from build123d import *

# Parameters (mm, degrees)
SKETCH7_W               = 120
SKETCH7_H               = 30
BOSS_EXTRUDE4_DEPTH     = 100
SKETCH8_W               = 20
SKETCH8_H               = 100
BOSS_EXTRUDE5_DEPTH     = 40
SKETCH9_W               = 100
SKETCH9_H               = 20
BOSS_EXTRUDE6_DEPTH     = 40
CUT_EXTRUDE2_DEPTH      = 99.261072461
CUT_EXTRUDE2_DEPTH_BACK = 40
SKETCH11_R              = 10
CUT_EXTRUDE3_DEPTH      = 120
SKETCH12_W              = 4
SKETCH12_H              = 16
SKETCH12_H_2            = 4
SKETCH12_W_2            = 16
SKETCH12_W_3            = 20
SKETCH12_H_3            = 20
BOSS_EXTRUDE7_DEPTH     = 30


with BuildPart() as part:
    # Sketch7 → Boss-Extrude4 (new body)
    with BuildSketch(Plane.XY):
        with Locations((0.090771558, -5.559757943)):
            Rectangle(SKETCH7_W, SKETCH7_H)
    extrude(amount=-BOSS_EXTRUDE4_DEPTH)

    # Sketch8 → Boss-Extrude5 (add)
    with BuildSketch(Plane(origin=(0, 9.440242057, 0), x_dir=(1, 0, 0), z_dir=(0, 1, 0))):
        with Locations((-49.909228442, 50)):
            Rectangle(SKETCH8_W, SKETCH8_H)
    extrude(amount=BOSS_EXTRUDE5_DEPTH)

    # Sketch9 → Boss-Extrude6 (add)
    with BuildSketch(Plane(origin=(0, 9.440242057, 0), x_dir=(1, 0, 0), z_dir=(0, 1, 0))):
        with Locations((10.090771558, 50)):
            Rectangle(SKETCH9_W, SKETCH9_H)
    extrude(amount=BOSS_EXTRUDE6_DEPTH)

    # Sketch10 → Cut-Extrude2 (cut, two sides: drawn at the far end of the back side and taken through both)
    with BuildSketch(Plane.XY.offset(-40).offset(-CUT_EXTRUDE2_DEPTH_BACK)):
        Polygon((-284.082083156, 147.109383943), (-39.909228442, 49.440242057), (60.090771558, 9.440242057), (304.263626273, -88.228899828), (499.601910045, 400.116809601), (-88.743799385, 635.455093373), align=None)
    extrude(amount=CUT_EXTRUDE2_DEPTH + CUT_EXTRUDE2_DEPTH_BACK, mode=Mode.SUBTRACT)

    # Sketch11 → Cut-Extrude3 (cut)
    with BuildSketch(Plane(origin=(60.090771558, 0, 0), x_dir=(0, 0, -1), z_dir=(1, 0, 0))):
        with Locations(Location((50, -5.559757943, 0), (0, 0, 90))):
            Circle(SKETCH11_R)
    extrude(amount=-CUT_EXTRUDE3_DEPTH, mode=Mode.SUBTRACT)

    # Sketch12 → Boss-Extrude7 (add)
    with BuildSketch(Plane.XZ.offset(20.559757943)):
        with Locations((-57.909228442, -12)):
            Rectangle(SKETCH12_W, SKETCH12_H)
        with Locations((-57.909228442, -2)):
            Rectangle(SKETCH12_W, SKETCH12_H_2)
        with Locations((-47.909228442, -2)):
            Rectangle(SKETCH12_W_2, SKETCH12_H_2)
        with Locations((48.090771558, -2)):
            Rectangle(SKETCH12_W_2, SKETCH12_H_2)
        with Locations((58.090771558, -12)):
            Rectangle(SKETCH12_W, SKETCH12_H)
        with Locations((58.090771558, -2)):
            Rectangle(SKETCH12_W, SKETCH12_H_2)
        with Locations((58.090771558, -88)):
            Rectangle(SKETCH12_W, SKETCH12_H)
        with Locations((58.090771558, -98)):
            Rectangle(SKETCH12_W, SKETCH12_H_2)
        with Locations((48.090771558, -98)):
            Rectangle(SKETCH12_W_2, SKETCH12_H_2)
        with Locations((-49.909228442, -98)):
            Rectangle(SKETCH12_W_3, SKETCH12_H_2)
        with Locations((-57.909228442, -90)):
            Rectangle(SKETCH12_W, SKETCH12_H_3)
    extrude(amount=BOSS_EXTRUDE7_DEPTH)


solid = part.part
Geometry check sheet. Reference: the model listing, model coordinates, mm. A direction names the side the tool comes from. Round coordinates to 2 decimals unless told otherwise and drop trailing zeros. Write each loop counter-clockwise with the first axis right and the second up, starting at its lowest first coordinate (ties: lowest second). Pieces come first, ordered by that corner, then holes.
Item 1: Section check D-D (x = -35). Record the boundary of the cut face in (y, z).
Determined:
outline: (-20.56, -100) - (9.44, -100) - (9.44, -60) - (47.48, -60) - (47.48, -40) - (9.44, -40) - (9.44, 0) - (-20.56, 0) - close; hole circle Ø20 at (-5.56, -50)
Item 2: Access from +Z, -Z, +X, -X, +Y, -Y to the whole of each face (thin tool, end or side, straight path). Record for faces 1 (the face through (40.091, -35, -2)), 2 (the face through (-2, 25, -60)), 3 (the face through (56.091, -35, -88)), 4 (the face through (-58, -35, -80)).
Determined:
face 1: +Z, -Z, -Y
face 2: -Z, +X, +Y
face 3: -Y
face 4: +X, -X, -Y
Item 3: Section check A-A (z = -50). Record the boundary of the cut face in (x, y), plus the area to 3 significant figures.
Determined:
outline: (-59.91, -20.56) - (60.09, -20.56) - (60.09, -15.56) - (-59.91, -15.56) - close; (-59.91, 4.44) - (60.09, 4.44) - (60.09, 9.44) - (-39.91, 49.44) - (-59.91, 49.44) - close
area: 4,000 mm2
Item 4: Section check B-B (y = -34). Record the boundary of the cut face in (x, z), plus the area to 3 significant figures.
Determined:
outline: (-59.91, -100) - (-39.91, -100) - (-39.91, -96) - (-55.91, -96) - (-55.91, -80) - (-59.91, -80) - close; (-59.91, -20) - (-55.91, -20) - (-55.91, -4) - (-39.91, -4) - (-39.91, 0) - (-59.91, 0) - close; (40.09, -100) - (60.09, -100) - (60.09, -80) - (56.09, -80) - (56.09, -96) - (40.09, -96) - close; (40.09, -4) - (56.09, -4) - (56.09, -20) - (60.09, -20) - (60.09, 0) - (40.09, 0) - close
area: 576 mm2
Item 5: Material ranges on line 1 along Z through (x, y) = (44.5, -39); line 2 along Z through (x, y) = (-22.5, 19); line 3 along Y through (x, z) = (-15, -16.5), recorded low to high.
Determined:
line 1: z = -100 to -96, -4 to 0
line 2: z = -60 to -40
line 3: y = -20.56 to 9.44
Item 6: Go/stop test with flat-tipped pins: pin 1 Ø12 at (y, z) = (32, -24) entering from +X; pin 2 Ø10 at (x, y) = (14, 19) entering from -Z; pin 3 Ø10 at (x, z) = (20, -87.5) entering from -Y; pin 4 Ø23 at (y, z) = (-5.56, -50) entering from +X. Record where each tip stops, or that it passes through.
Determined:
pin 1: stops at x = -39.91
pin 2: stops at z = -60
pin 3: stops at y = -20.56
pin 4: stops at x = 60.09
Item 7: Mould release check, pull along Z, two halves, no side actions. Record for faces 5 (the face through (-48, -35, -96)), 6 (the face through (9.39, 29.72, -50.14)), 7 (the face through (-2, 25, -40)): +Z half, -Z half, draft (parallel to the pull), parting line (faces both ways), or undercut.
Determined:
face 5: undercut
face 6: draft
face 7: +Z half
Item 8: Section check C-C (y = -5.5). Record the boundary of the cut face in (x, z), plus the area to 3 significant figures.
Determined:
outline: (-59.91, -100) - (60.09, -100) - (60.09, -60) - (-59.91, -60) - close; (-59.91, -40) - (60.09, -40) - (60.09, 0) - (-59.91, 0) - close
area: 9,600 mm2
